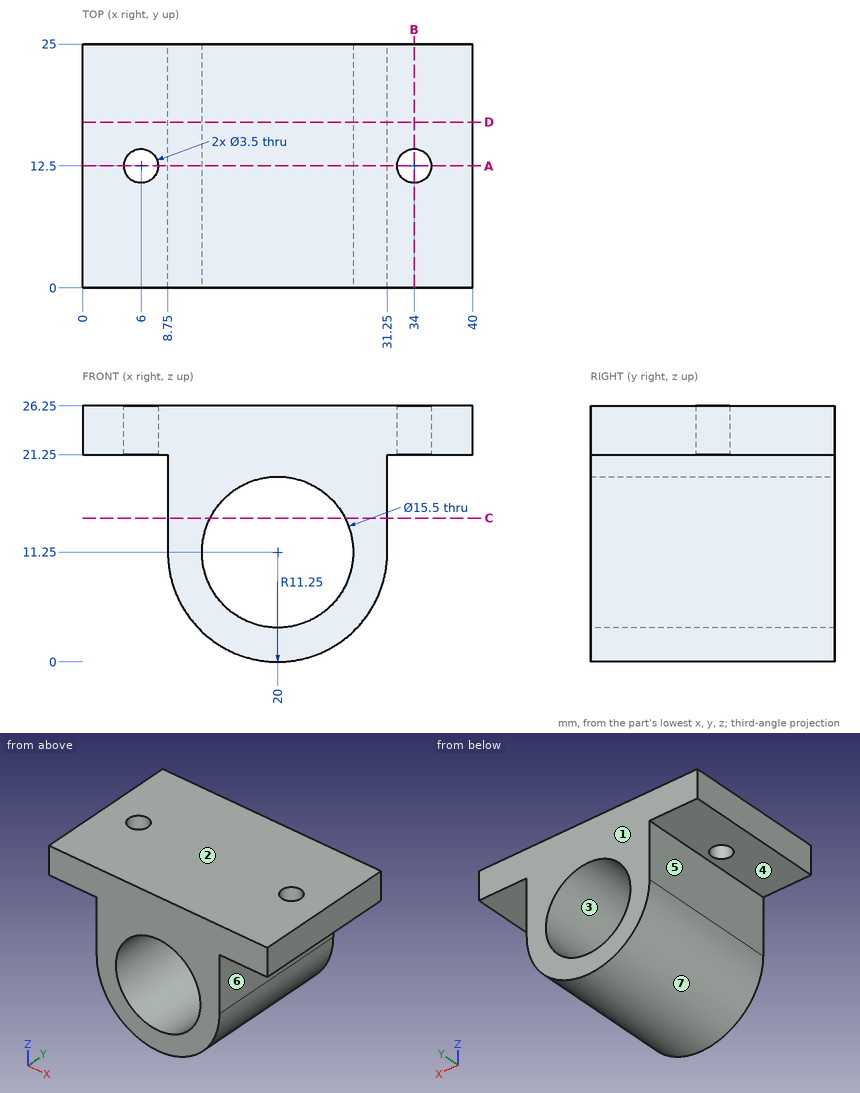
Input: dimensioned drawing with shaded views. Units: mm. Origin: part minimum x, y, z. A direction names the side the tool comes from. Give positions to 0.01 mm unless a question says otherwise; leave off trailing zeros. Order: outer loops, then holes, each group sorted by start corner. A loop starts at its lowest first (then second) coordinate and runs counter-clockwise, first axis right, second up. Notation, with made-up numbers: (64, -3.5) -> (92, -3.5) arc R33 ccw to (92, 30.5) -> close; hole circle Ø8 at (89.25, 44). An arc over 180 degrees is marked (long way). Answer as a JSON object with one key per item and string values.
Q1. Section B-B (x = 34). Output: boundary loops of the cut face in (y, z), plus the area to 4 significant figures.
Entries:
{"outline": "(0, 21.25) -> (10.75, 21.25) -> (10.75, 26.25) -> (0, 26.25) -> close; (14.25, 21.25) -> (25, 21.25) -> (25, 26.25) -> (14.25, 26.25) -> close", "area": "107.5 mm^2"}
Q2. Section D-D (y = 17). Output: boundary loops of the cut face in (x, z).
Entries:
{"outline": "(0, 21.25) -> (8.75, 21.25) -> (8.75, 11.25) arc R11.25 ccw to (31.25, 11.25) -> (31.25, 21.25) -> (40, 21.25) -> (40, 26.25) -> (0, 26.25) -> close; hole circle Ø15.5 at (20, 11.25)"}
Q3. Draft query along Z for the marked faces 1, 2, 3 and 4. Return one class per face: released by +Z, released by -Z, zero draft, split by the parting line, or undercut.
Entries:
{"face 1": "zero draft", "face 2": "released by +Z", "face 3": "undercut", "face 4": "released by -Z"}
Q4. Material intervals for probe 1 along Y at (x, z) = (34, 22.7); probe 2 along Z at (x, y) = (32.5, 11.25); probe 3 along X at (y, z) = (11, 11.25), sorted ascending.
Entries:
{"probe 1": "y = 0 to 10.75, 14.25 to 25", "probe 2": "z = 21.25 to 26.25", "probe 3": "x = 8.75 to 12.25, 27.75 to 31.25"}
Q5. First-contact query: pin 1 (12.5 mm diameter, centred on x = 20, z = 11.25, fed in from +Y); pin 2 (1.5 mm diameter, centred on y = 10.5, z = 6.5, fed in from +X); pin 3 (1 mm diameter, centred on x = 9.5, y = 3, fed in from -Z); pin 4 (11 mm diameter, centred on y = 8.5, z = 15.5, fed in from -X). Flat tips, straight axial feed; report the tip coordinate or a pass-through.
Entries:
{"pin 1": "passes through", "pin 2": "stops at x = 30.51", "pin 3": "stops at z = 6.1", "pin 4": "stops at x = 8.75"}
Q6. Access query for the marked faces 5, 6 and 7. Directions: +Z, -Z, +X, -X, +Y, -Y. A direction counts if a zero-diameter tool reaches every point of the face in a straight line with its end or side. Return the directions, or none.
Entries:
{"face 5": "-Z, -X, +Y, -Y", "face 6": "-Z, +X, +Y, -Y", "face 7": "-Z, +Y, -Y"}
Q7. Section A-A (y = 12.5). Output: boundary loops of the cut face in (x, z), plus the area to 3 significant figures.
Entries:
{"outline": "(0, 21.25) -> (4.25, 21.25) -> (4.25, 26.25) -> (0, 26.25) -> close; (7.75, 21.25) -> (8.75, 21.25) -> (8.75, 11.25) arc R11.25 ccw to (31.25, 11.25) -> (31.25, 21.25) -> (32.25, 21.25) -> (32.25, 26.25) -> (7.75, 26.25) -> close; (35.75, 21.25) -> (40, 21.25) -> (40, 26.25) -> (35.75, 26.25) -> close; hole circle Ø15.5 at (20, 11.25)", "area": "400 mm^2"}
Q8. Section C-C (z = 14.75). Output: boundary loops of the cut face in (x, y).
Entries:
{"outline": "(8.75, 0) -> (13.09, 0) -> (13.09, 25) -> (8.75, 25) -> close; (26.91, 0) -> (31.25, 0) -> (31.25, 25) -> (26.91, 25) -> close"}
